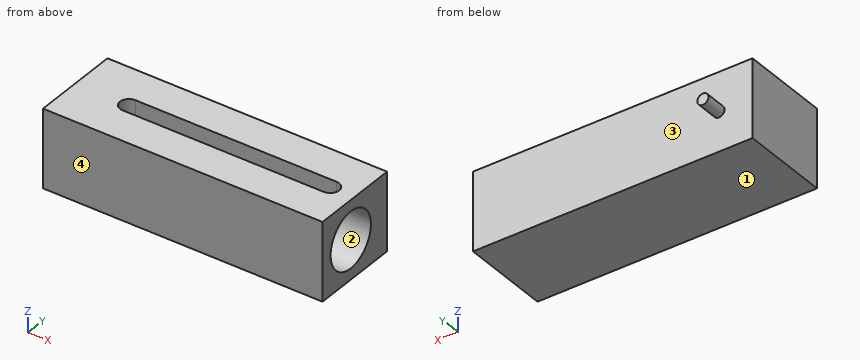
from build123d import *

# Parameters (mm, degrees)
SKETCH1_W               = 250
SKETCH1_H               = 70
BOSS_EXTRUDE1_DEPTH     = 80
SKETCH2_R               = 25
CUT_EXTRUDE1_DEPTH      = 210
CUT_EXTRUDE2_REACH      = 166.088
CUT_EXTRUDE2_END_RADIUS = 25
SKETCH4_R               = 5
BOSS_EXTRUDE2_DEPTH     = 20


with BuildPart() as part:
    # Sketch1 → Boss-Extrude1 (new body)
    with BuildSketch(Plane(origin=(0, 0, 0), x_dir=(1, 0, 0), z_dir=(0, 1, 0))):
        Rectangle(SKETCH1_W, SKETCH1_H)
    extrude(amount=BOSS_EXTRUDE1_DEPTH)

    # Sketch2 → Cut-Extrude1 (cut)
    with BuildSketch(Plane(origin=(125, 0, 0), x_dir=(0, 0, -1), z_dir=(1, 0, 0))):
        with Locations((0, 35)):
            Circle(SKETCH2_R)
    extrude(amount=-CUT_EXTRUDE1_DEPTH, mode=Mode.SUBTRACT)

    # Cut-Extrude2: up to this cylinder (the profile starts outside it)
    cut_extrude2_end = Plane(origin=(13, 35, 0), z_dir=(1, 0, 0)) * Cylinder(CUT_EXTRUDE2_END_RADIUS, 383.176, mode=Mode.PRIVATE)
    # Sketch3 → Cut-Extrude2 (cut, up to the surface)
    with BuildSketch(Plane.XY.offset(35), mode=Mode.PRIVATE) as cut_extrude2_sk1:
        with BuildLine():
            Line((103, 32), (-77, 32))
            ThreePointArc((-77, 32), (-85, 40), (-77, 48))
            Line((-77, 48), (103, 48))
            ThreePointArc((103, 48), (111, 40), (103, 32))
        make_face()
    cut_extrude2_tool1 = extrude(cut_extrude2_sk1.sketch, amount=-CUT_EXTRUDE2_REACH, mode=Mode.PRIVATE) - cut_extrude2_end
    add(cut_extrude2_tool1.solids().sort_by_distance((13, 40, 35))[0], mode=Mode.SUBTRACT)

    # Sketch4 → Boss-Extrude2 (add)
    with BuildSketch(Plane(origin=(0, 80, 0), x_dir=(1, 0, 0), z_dir=(0, 1, 0))):
        with Locations(Location((-95.026953026, 0, 0), (0, 0, 270))):
            Circle(SKETCH4_R)
    extrude(amount=BOSS_EXTRUDE2_DEPTH)


solid = part.part
Input: part model. Units: mm. Frame: model coordinates. Face numbers are marked on the shaded views. Give positions to 0.01 mm unless a question says otherwise; leave off trailing zeros. Write each loop counter-clockwise with the first axis right and the second up, starting at its lowest first coordinate (ties: lowest second). Pieces come first, ordered by that corner, then holes.
Q1. Pull-direction query (Y, two-part tool) for the marked faces 1, 2, 3 and 4; classes: pulls with the +Y half, pulls with the -Y half, needs draft (parallel to the pull), parting line crosses it, or undercut.
Q2. Section A-A, the plane y = 44. Output: boundary loops of the cut face in (x, z).
Q3. Section D-D, the plane z = 14. Output: boundary loops of the cut face in (x, y).
Q4. Section B-B, the plane x = -67. Output: boundary loops of the cut face in (y, z), plus the area to 3 significant figures.
Q5. Section C-C, the plane z = 0. Output: boundary loops of the cut face in (x, y), plus the area to 3 significant figures.
Q6. Material intervals for probe 1 along Y at (x, z) = (0, 0); probe 2 along Z at (x, y) = (-32, 35); probe 3 along X at (y, z) = (12.5, 10.5), sorted ascending.
Q7. First-contact query: P1, Ø8, axis at x = -31, z = -24, coming from the +Y side. Flat tip, straight axial feed; report the tip coordinate or a pass-through.
Filled in:
1. face 1: needs draft
1. face 2: undercut
1. face 3: pulls with the +Y half
1. face 4: pulls with the -Y half
2. outline: (-125, -35) - (125, -35) - (125, -23.32) - (-85, -23.32) - (-85, 23.32) - (-83.93, 23.32) - (-83.93, 35) - (-125, 35) - close; (109.93, 23.32) - (125, 23.32) - (125, 35) - (109.93, 35) - close
3. outline: (-125, 0) - (125, 0) - (125, 14.29) - (-85, 14.29) - (-85, 55.71) - (125, 55.71) - (125, 80) - (-125, 80) - close
4. outline: (0, -35) - (80, -35) - (80, 35) - (48, 35) - (48, 21.35) arc R25 cw (long way) to (32, 24.82) - (32, 35) - (0, 35) - close
4. area: 3,460 mm2
5. outline: (-125, 0) - (125, 0) - (125, 10) - (-85, 10) - (-85, 60) - (125, 60) - (125, 80) - (-90.03, 80) - (-90.03, 100) - (-100.03, 100) - (-100.03, 80) - (-125, 80) - close
5. area: 9,700 mm2
6. probe 1: y = 0 to 10, 60 to 80
6. probe 2: z = -35 to -25
6. probe 3: x = -125 to -85
7. P1: stops at y = 80
